Part model, mm, in its own coordinate system. A direction names the side the tool comes from. Give positions to 0.01 mm unless a question says otherwise; leave off trailing zeros. Order: outer loops, then holes, each group sorted by start corner. A loop starts at its lowest first (then second) coordinate and runs counter-clockwise, first axis right, second up. Notation, with made-up numbers: (58.5, 11.5) - (80.5, 11.5) arc R26 cw to (80.5, 45.5) - close; hole circle Ø5 at (80.5, -29.75). An arc over 180 degrees is marked (long way). Use one line per item in the form item = value. Start each with the question number.
1. Drill centre lines: line 1 (X direction, y = 76.75, z = 34); line 2 (X direction, y = -36, z = 173.5); line 3 (Y direction, x = 40.5, z = 128). Where is each one in solid material? Low to high.
2. Tool access for faces 5 (the face through (-1, -1, 4)), 6 (the face through (-4.213, 76.37, 23.839)): list every direction of +Z, -Z, +X, -X, +Y, -Y with a clear straight run to the whole face (end or side of a thin tool).
3. Band-saw the part on D-D, the plane z = 183. List the corners of the cut face in (x, y), plus the area to 3 significant figures.
4. Band-saw the part on C-C, the plane y = -13.5. List the corners of the cut face in (x, z), plus the area to 3 significant figures.
5. Band-saw the part on A-A, the plane z = 34. List the corners of the cut face in (x, y).
6. Pull direction X, two halves, no side cores. Call faces 1 (the face through (-4.213, -76.43, 23.839)), 2 (the face through (-78.8, -1, 101)), 3 (the face through (-1, 74.25, 103)), 4 (the face through (-1, 78.55, 101)): +X half, -X half, draft (parallel to the pull), parting line (faces both ways), or undercut.
7. Band-saw the part on B-B, the plane x = 0. List the corners of the cut face in (y, z).
from build123d import *

# Parameters (mm, degrees)
CROQUIS1_W              = 157.6
CROQUIS1_H              = 157.1
CROQUIS1_W_2            = 149
CROQUIS1_H_2            = 148.5
SALIENTE_EXTRUIR1_DEPTH = 204.5
CROQUIS2_W              = 4
CROQUIS2_H              = 157.1
SALIENTE_EXTRUIR2_DEPTH = 149
CROQUIS3_R              = 11
CORTAR_EXTRUIR1_DEPTH   = 270.648104017


with BuildPart() as part:
    # Croquis1 → Saliente-Extruir1 (new body)
    with BuildSketch(Plane.XY):
        Rectangle(CROQUIS1_W, CROQUIS1_H)
        Rectangle(CROQUIS1_W_2, CROQUIS1_H_2, mode=Mode.SUBTRACT)
    extrude(amount=SALIENTE_EXTRUIR1_DEPTH)

    # Croquis2 → Saliente-Extruir2 (add)
    with BuildSketch(Plane(origin=(-74.5, 0, 0), x_dir=(0, 0, -1), z_dir=(1, 0, 0))):
        with Locations((-2, 0)):
            Rectangle(CROQUIS2_W, CROQUIS2_H)
    extrude(amount=SALIENTE_EXTRUIR2_DEPTH)

    # Croquis3 → Cortar-Extruir1 (cut, through all)
    with BuildSketch(Plane.XZ.offset(78.55)):
        with Locations(Location((0, 34, 0), (0, 0, 270))):
            Circle(CROQUIS3_R)
    extrude(amount=-CORTAR_EXTRUIR1_DEPTH, mode=Mode.SUBTRACT)


solid = part.part
From the geometry:
q1.line_1 = -78.8 to -11, 11 to 78.8
q1.line_2 = -78.8 to -74.5, 74.5 to 78.8
q1.line_3 = -78.55 to -74.25, 74.25 to 78.55
q2.face_5 = +Z
q2.face_6 = +Y, -Y
q3.outline = (-78.8, -78.55) - (78.8, -78.55) - (78.8, 78.55) - (-78.8, 78.55) - close; hole (-74.5, -74.25) - (74.5, -74.25) - (74.5, 74.25) - (-74.5, 74.25) - close
q3.area = 2,630 mm²
q4.outline = (-78.8, 0) - (78.8, 0) - (78.8, 204.5) - (74.5, 204.5) - (74.5, 4) - (-74.5, 4) - (-74.5, 204.5) - (-78.8, 204.5) - close
q4.area = 2,350 mm²
q5.outline = (-78.8, -78.55) - (-11, -78.55) - (-11, -74.25) - (-74.5, -74.25) - (-74.5, 74.25) - (-11, 74.25) - (-11, 78.55) - (-78.8, 78.55) - close; (11, -78.55) - (78.8, -78.55) - (78.8, 78.55) - (11, 78.55) - (11, 74.25) - (74.5, 74.25) - (74.5, -74.25) - (11, -74.25) - close
q6.face_1 = undercut
q6.face_2 = -X half
q6.face_3 = undercut
q6.face_4 = draft
q7.outline = (-78.55, 0) - (78.55, 0) - (78.55, 23) - (74.25, 23) - (74.25, 4) - (-74.25, 4) - (-74.25, 23) - (-78.55, 23) - close; (-78.55, 45) - (-74.25, 45) - (-74.25, 204.5) - (-78.55, 204.5) - close; (74.25, 45) - (78.55, 45) - (78.55, 204.5) - (74.25, 204.5) - close
